from build123d import *

# Parameters (mm, degrees)
SKETCH1_W           = 50
SKETCH1_H           = 25
BOSS_EXTRUDE1_DEPTH = 4
CHAMFER1_SIZE       = 4
CHAMFER1_SIZE2      = 2.309401077
SKETCH2_W           = 10
SKETCH2_H           = 10
BOSS_EXTRUDE2_DEPTH = 5.5
CUT_EXTRUDE1_REACH  = 37.781
SKETCH3_W           = 0.8
SKETCH3_H           = 0.8
LPATTERN1_COUNT     = 16
LPATTERN1_PITCH     = 2
CHAMFER2_SIZE       = 1
CHAMFER2_SIZE2      = 0.577350269


with BuildPart() as part:
    # Sketch1 → Boss-Extrude1 (new body)
    with BuildSketch(Plane.XY):
        Rectangle(SKETCH1_W, SKETCH1_H)
    extrude(amount=BOSS_EXTRUDE1_DEPTH)

    # Chamfer1
    chamfer1_edges = [part.edges().sort_by_distance(p)[0] for p in [
        (25, 0, 0),
    ]]
    chamfer1_side = [part.faces().sort_by_distance(p)[0] for p in [
        (0, 0, 0),
    ]]
    chamfer(chamfer1_edges, length=CHAMFER1_SIZE, length2=CHAMFER1_SIZE2, reference=chamfer1_side[0])

    # Sketch2 → Boss-Extrude2 (add)
    with BuildSketch(Plane(origin=(0, 0, 0), x_dir=(-1, 0, 0), z_dir=(0, 0, -1))):
        with Locations((-10, 0)):
            Rectangle(SKETCH2_W, SKETCH2_H)
    extrude(amount=BOSS_EXTRUDE2_DEPTH)

    # Sketch3 → Cut-Extrude1 (cut, up to next)
    with BuildSketch(Plane(origin=(0, 12.5, 0), x_dir=(1, 0, 0), z_dir=(0, 1, 0)), mode=Mode.PRIVATE) as cut_extrude1_sk1:
        with Locations((24, -4)):
            Rectangle(SKETCH3_W, SKETCH3_H)
    cut_extrude1_tool1 = extrude(cut_extrude1_sk1.sketch, amount=-CUT_EXTRUDE1_REACH, mode=Mode.PRIVATE) & part.part
    cut_extrude1 = cut_extrude1_tool1.solids().sort_by_distance((24, 12.5, 4))[0]
    add(cut_extrude1, mode=Mode.SUBTRACT)

    # LPattern1: Cut-Extrude1 ×16
    with Locations(*[(-i * LPATTERN1_PITCH, 0, 0) for i in range(1, LPATTERN1_COUNT)]):
        add(cut_extrude1, mode=Mode.SUBTRACT)

    # Chamfer2
    chamfer2_edges = [part.edges().sort_by_distance(p)[0] for p in [
        (-25, 0, 0),
    ]]
    chamfer2_side = [part.faces().sort_by_distance(p)[0] for p in [
        (-3.142857143, 0, 0),
    ]]
    chamfer(chamfer2_edges, length=CHAMFER2_SIZE, length2=CHAMFER2_SIZE2, reference=chamfer2_side[0])


solid = part.part
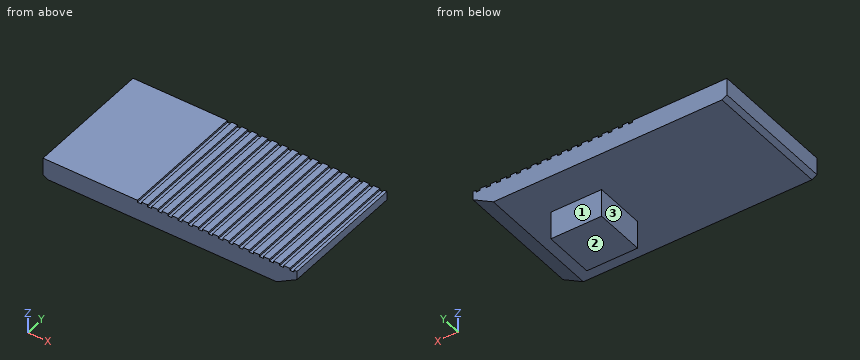
Can you work these out from the model? Positions are in its coordinate system, mm. Face numbers are marked on the shaded views. A direction names the side the tool comes from. Coordinates: 2 decimals unless noted, no trailing zeros. Loops run counter-clockwise (first coordinate to the right, second up) from the corner with the lowest first, then second, coordinate; pieces in that order, holes last. Notation, with made-up numbers: (47.5, 33.25) - (55.5, 33.25) arc R29 ccw to (55.5, 61.25) - close; hole circle Ø8 at (-16, 3.5). An arc over 180 degrees is marked (long way). Put each result on its own line as item: value. Start each with the question number.
Item 1: For pin 1 (0.6 mm diameter, centred on x = 4, y = -5.5, fed in from +Z); pin 2 (1 mm diameter, centred on x = -15.5, y = 8, fed in from -Z); pin 3 (3 mm diameter, centred on y = -2.5, z = -2, fed in from +X), each with a flat end and sliding along its axis, tell me the tip position at first contact or that it passes through.
Item 2: Which directions (+Z, -Z, +X, -X, +Y, -Y) give clear straight access to the entire face, cutting with the end or side of a thin tool? Please do the marked faces 1, 2 and 3.
Item 3: Suppose I cut it at C-C (x = -17.5). Please give me the cut outline in (y, z), and give its area (3 significant figures).
Item 4: Suppose I cut it at A-A (x = 11). Please give me the cut outline in (y, z).
Item 5: Suppose I cut it at B-B (z = -1). Please give me the cut outline in (x, y), and give its area (3 significant figures).
Item 6: If I drill on line 1 along X through (y, z) = (0.25, -4.75); line 2 along Z through (x, y) = (-10, -9.75); line 3 along Y through (x, z) = (10, -2.75), over which ranges is the centre line in solid material (lowest first)?
Here are the results:
1. pin 1: z = 3.6
1. pin 2: z = 0
1. pin 3: x = 15
2. face 1: -Z, +X, -X, +Y
2. face 2: -Z, +X, -X, +Y, -Y
2. face 3: -Z, -X, +Y, -Y
3. outline: (-12.5, 0) - (12.5, 0) - (12.5, 4) - (-12.5, 4) - close
3. area: 100 mm²
4. outline: (-12.5, 0) - (-5, 0) - (-5, -5.5) - (5, -5.5) - (5, 0) - (12.5, 0) - (12.5, 4) - (-12.5, 4) - close
5. outline: (5, -5) - (15, -5) - (15, 5) - (5, 5) - close
5. area: 100 mm²
6. line 1: 5 to 15
6. line 2: 0 to 4
6. line 3: -5 to 5
